from build123d import *

# Parameters (mm, degrees)
F0_W     = 285
F0_H     = 200
F1_DEPTH = 5
F2_W     = 225
F2_H     = 170
F3_DEPTH = 25
F4_R     = 1.5
F5_DEPTH = 25


with BuildPart() as f1:
    # F0 (on Front) → F1 (new body)
    with BuildSketch(Plane.XZ):
        Rectangle(F0_W, F0_H)
    extrude(amount=F1_DEPTH)

    # F2 (on face) → F3 (cut)
    with BuildSketch(Plane.XZ.offset(5)):
        with Locations((0, -15)):
            Rectangle(F2_W, F2_H)
    extrude(amount=-F3_DEPTH, mode=Mode.SUBTRACT)

    # F4 (on face) → F5 (cut)
    with BuildSketch(Plane.XZ.offset(5)):
        with Locations((-10, 85)):
            Circle(F4_R)
        with Locations((10, 85)):
            Circle(F4_R)
    extrude(amount=-F5_DEPTH, mode=Mode.SUBTRACT)


solid = f1.part
Here's how the part is built. I have some questions about the finished solid (model axes, mm). Give positions to 0.01 mm unless a question says otherwise; leave off trailing zeros. Order: outer loops, then holes, each group sorted by start corner. A loop starts at its lowest first (then second) coordinate and runs counter-clockwise, first axis right, second up. Notation, with made-up numbers: M 89.25,28.5 L 125.25,28.5 A22 ccw 125.25,41.5 Z; hole C -36.75,-25.5 d6. An arc over 180 degrees is marked long. Answer as a JSON object with one key per item and string values. Group by question number.
1) Suppose I cut it at A-A, the plane z = -67.5. Write out the boundary of the cut face in (x, y).
2) Suppose I cut it at B-B, the plane y = -2.2. Write out the boundary of the cut face in (x, z).
3) Suppose I cut it at C-C, the plane x = -67. Write out the boundary of the cut face in (y, z), plus the area to 3 significant figures.
4) Please list where these lines run through material, in increasing order: L1, parallel to X at y = -3.1, z = 85; L2, parallel to X at y = -2.55, z = 46.5; L3, parallel to Z at x = -10, y = -3.3. Write a range as [from, to].
5) I'm going to push a flat-ended pin straight in: pin 1 Ø1 at (x, y) = (3, -2.5) entering from -Z. Where does the tip first touch, or does it pass through?
Results found:
{
 "1": {"outline": "M -142.5,-5 L -112.5,-5 L -112.5,0 L -142.5,0 Z; M 112.5,-5 L 142.5,-5 L 142.5,0 L 112.5,0 Z"},
 "2": {"outline": "M -142.5,-100 L -112.5,-100 L -112.5,70 L 112.5,70 L 112.5,-100 L 142.5,-100 L 142.5,100 L -142.5,100 Z; hole C -10,85 d3; hole C 10,85 d3"},
 "3": {"outline": "M -5,70 L 0,70 L 0,100 L -5,100 Z", "area": "150 mm²"},
 "4": {"L1": "[-142.5, -11.5], [-8.5, 8.5], [11.5, 142.5]", "L2": "[-142.5, -112.5], [112.5, 142.5]", "L3": "[70, 83.5], [86.5, 100]"},
 "5": {"pin 1": "z = 70"}
}
